Source: CAD feature listing. Evaluate the final solid. Frame: model axes, mm. A direction names the side the tool comes from. Give positions to 0.01 mm unless a question says otherwise; leave off trailing zeros. Order: outer loops, then holes, each group sorted by start corner. A loop starts at its lowest first (then second) coordinate and runs counter-clockwise, first axis right, second up. Notation, with made-up numbers: M -32,-9.5 L 23,-9.5 A36 ccw 23,27.5 Z; hole C 7,-32.75 d6. An arc over 180 degrees is marked long. Answer as a JSON object with one key per item and string values. Group by question number.
1. Set-up query: faces 1 (the flat face through (-18, -11, -3.81)), 2 (the flat face through (-44.45, 2, 5)), 3 (the cylindrical face through (0.71, 145.73, -7.08)). Return all of +Z, -Z, +X, -X, +Y, -Y with unobstructed straight access to the full face (end or side cutting, diameter ignored); none if empty.
2. Material intervals for L1, parallel to X at y = -11.5, z = -3; L2, parallel to X at y = -71, z = 4; L3, parallel to X at y = -40, z = 6, sorted ascending. Write a range as [from, to].
3. Pull-direction query (X, two-part tool) for faces 4 (the cylindrical face through (50.174, 145.827, 6.98)), 5 (the flat face through (44.45, 2, 5)), 6 (the flat face through (57.15, -5, 0)); classes: +X half, -X half, draft (parallel to the pull), parting line (faces both ways), or undercut.
4. Section query B-B (y = -0.5). Output: boundary loops of the cut face in (x, z) (3 decimals).
5. Pin query (flat end, axial travel): P1, Ø1, axis at x = 29, z = 3.5, coming from the +Y side; P2, Ø2.5, axis at y = -15.5, z = 4, coming from the -X side; P3, Ø1.9, axis at x = -18.5, y = -10, coming from the +Z side. Return the tip coordinate at first contact, or that it passes through.
from build123d import *

# Parameters (mm, degrees)
SKETCH1_W           = 114.3
SKETCH1_H           = 295.275
BOSS_EXTRUDE1_DEPTH = 8.89
SKETCH2_R           = 3.175
CUT_EXTRUDE1_DEPTH  = 12.7
SKETCH3_W           = 5.08
SKETCH3_H           = 8.255
CUT_EXTRUDE2_DEPTH  = 296.275
FILLET1_R           = 6.35
SKETCH5_R           = 7.9375
CUT_EXTRUDE4_DEPTH  = 18.78


with BuildPart() as part:
    # Sketch1 → Boss-Extrude1 (new body, symmetric)
    with BuildSketch(Plane.XY):
        Rectangle(SKETCH1_W, SKETCH1_H)
    extrude(amount=BOSS_EXTRUDE1_DEPTH, both=True)

    # Sketch2 → Cut-Extrude1 (cut)
    with BuildSketch(Plane.XY.offset(8.89)):
        with Locations((0, -11.1125)):
            Circle(SKETCH2_R)
        with Locations((-17.526, -11.1125)):
            Circle(SKETCH2_R)
        with Locations((17.526, -11.1125)):
            Circle(SKETCH2_R)
    extrude(amount=-CUT_EXTRUDE1_DEPTH, mode=Mode.SUBTRACT)

    # Sketch3 → Cut-Extrude2 (cut, through all)
    with BuildSketch(Plane(origin=(0, 147.6375, 0), x_dir=(1, 0, 0), z_dir=(0, 1, 0))):
        with Locations((-46.99, -4.7625)):
            Rectangle(SKETCH3_W, SKETCH3_H)
    cut_extrude2 = extrude(amount=-CUT_EXTRUDE2_DEPTH, mode=Mode.SUBTRACT)

    # Mirror1: Cut-Extrude2 across plane
    add(cut_extrude2.mirror(Plane(origin=(0, 0, 0), x_dir=(0, 0, 1), z_dir=(1, 0, 0))), mode=Mode.SUBTRACT)

    # Fillet1
    fillet1_edges = [part.edges().sort_by_distance(p)[0] for p in [
        (-57.15, 0, 8.89),
        (-53.34, 147.6375, 8.89),
        (57.15, 0, 8.89),
        (0, 147.6375, 8.89),
        (-57.15, 0, -8.89),
        (0, 147.6375, -8.89),
        (57.15, 0, -8.89),
        (53.34, 147.6375, 8.89),
        (-57.15, 147.6375, 0),
        (57.15, 147.6375, 0),
    ]]
    fillet(fillet1_edges, radius=FILLET1_R)

    # Sketch5 → Cut-Extrude4 (cut, through all)
    with BuildSketch(Plane.XY.offset(8.89)):
        with Locations((0, -65.0875)):
            Circle(SKETCH5_R)
    extrude(amount=-CUT_EXTRUDE4_DEPTH, mode=Mode.SUBTRACT)


solid = part.part
Answer sheet:
{
 "1": {"face 1": "+Z", "face 2": "+Z, +Y, -Y", "face 3": "-Z, +X, -X, +Y"},
 "2": {"L1": "[-57.13, -20.68], [-14.37, -3.15], [3.15, 14.37], [20.68, 57.13]", "L2": "[-56.98, -49.53], [-44.45, -5.3], [5.3, 44.45], [49.53, 56.98]", "L3": "[-56.12, -49.53], [-44.45, 44.45], [49.53, 56.12]"},
 "3": {"face 4": "draft", "face 5": "undercut", "face 6": "+X half"},
 "4": {"outline": "M -57.15,-2.54 A6.35 ccw -50.8,-8.89 L 50.8,-8.89 A6.35 ccw 57.15,-2.54 L 57.15,2.54 A6.35 ccw 50.8,8.89 L 49.53,8.89 L 49.53,0.635 L 44.45,0.635 L 44.45,8.89 L -44.45,8.89 L -44.45,0.635 L -49.53,0.635 L -49.53,8.89 L -50.8,8.89 A6.35 ccw -57.15,2.54 Z"},
 "5": {"P1": "y = 147.62", "P2": "x = -57.15", "P3": "z = -3.81"}
}
